```python
from build123d import *

# Parameters (mm, degrees)
BOSS_EXTRUDE1_DEPTH      = 9
BOSS_EXTRUDE1_DEPTH_BACK = 9
SKETCH1_R                = 1.625
SKETCH2_OUTSIDE_W        = 79.846
SKETCH2_OUTSIDE_H        = 80.774
SKETCH2_OUTSIDE_R        = 3
CUT_EXTRUDE1_DEPTH       = 19.574175621
CUT_EXTRUDE1_DRAFT       = -60
SKETCH3_OUTSIDE_W        = 79.846
SKETCH3_OUTSIDE_H        = 80.774
SKETCH3_OUTSIDE_R        = 3
CUT_EXTRUDE2_DEPTH       = 19.574175621
CUT_EXTRUDE2_DRAFT       = -60
CHAMFER1_SIZE            = 0.25


with BuildPart() as part:
    # Sketch1 → Boss-Extrude1 (new, two sides: drawn at the far end of the back side and taken through both)
    with BuildSketch(Plane.XY.offset(-BOSS_EXTRUDE1_DEPTH_BACK)):
        Polygon((0, 3.464101615), (-3, 1.732050808), (-3, -1.732050808), (0, -3.464101615), (3, -1.732050808), (3, 1.732050808), align=None)
        Circle(SKETCH1_R, mode=Mode.SUBTRACT)
    extrude(amount=BOSS_EXTRUDE1_DEPTH + BOSS_EXTRUDE1_DEPTH_BACK)


with BuildPart() as cut_extrude1_tool:
    # Sketch2 outside → Cut-Extrude1 (with draft: the straight prism first)
    with BuildSketch(Plane(origin=(0, 0, -9), x_dir=(-1, 0, 0), z_dir=(0, 0, -1))):
        Rectangle(SKETCH2_OUTSIDE_W, SKETCH2_OUTSIDE_H)
        Circle(SKETCH2_OUTSIDE_R, mode=Mode.SUBTRACT)
    extrude(amount=-CUT_EXTRUDE1_DEPTH)
    # Cut-Extrude1: the draft: its side faces are tilted about the plane it starts from
    cut_extrude1_sides = [cut_extrude1_tool.faces().sort_by_distance(p)[0] for p in [
        (0, -40.387, 0.787087811),
        (-39.923, 0, 0.787087811),
        (0, 40.387, 0.787087811),
        (39.923, 0, 0.787087811),
        (3, 0, 0.787087811),
    ]]
    draft(cut_extrude1_sides, Plane(origin=(0, 0, -9), x_dir=(-1, 0, 0), z_dir=(0, 0, -1)), CUT_EXTRUDE1_DRAFT)


with BuildPart() as part_1:
    add(part.part)

    # Cut-Extrude1: cut by cut_extrude1_tool
    add(cut_extrude1_tool.part, mode=Mode.SUBTRACT)


with BuildPart() as cut_extrude2_tool:
    # Sketch3 outside → Cut-Extrude2 (with draft: the straight prism first)
    with BuildSketch(Plane.XY.offset(9)):
        Rectangle(SKETCH3_OUTSIDE_W, SKETCH3_OUTSIDE_H)
        Circle(SKETCH3_OUTSIDE_R, mode=Mode.SUBTRACT)
    extrude(amount=-CUT_EXTRUDE2_DEPTH)
    # Cut-Extrude2: the draft: its side faces are tilted about the plane it starts from
    cut_extrude2_sides = [cut_extrude2_tool.faces().sort_by_distance(p)[0] for p in [
        (0, -40.387, -0.787087811),
        (39.923, 0, -0.787087811),
        (0, 40.387, -0.787087811),
        (-39.923, 0, -0.787087811),
        (-3, 0, -0.787087811),
    ]]
    draft(cut_extrude2_sides, Plane.XY.offset(9), CUT_EXTRUDE2_DRAFT)


with BuildPart() as part_2:
    add(part_1.part)

    # Cut-Extrude2: cut by cut_extrude2_tool
    add(cut_extrude2_tool.part, mode=Mode.SUBTRACT)

    # Chamfer1
    chamfer1_edges = [part_2.edges().sort_by_distance(p)[0] for p in [
        (-1.625, 0, -9),
        (-1.625, 0, 9),
    ]]
    chamfer(chamfer1_edges, length=CHAMFER1_SIZE)


solid = part_2.part
```
For this review, take the finished solid that the model builds, in its own axes (mm). Round coordinates to 2 decimals unless told otherwise and drop trailing zeros. Order: outer loops, then holes, each group sorted by start corner. A loop starts at its lowest first (then second) coordinate and runs counter-clockwise, first axis right, second up.
Q1. Insertion check: P1, Ø2.5, axis at x = 0, y = 0, coming from the +Z side. The pin has a flat end and moves straight along its axis. Give the tip position at first contact, or say it passes through.
Findings below:
P1: passes through
Q2. Wall thickness on line 1 (Y direction, x = -0.75, z = 0.5); line 2 (X direction, y = 0.5, z = 2.25); line 3 (Y direction, x = 0.5, z = -2.25): over which ranges is each line inside the solid? List them lowest first.
Findings below:
line 1: y = -3.03 to -1.44, 1.44 to 3.03
line 2: x = -3 to -1.55, 1.55 to 3
line 3: y = -3.18 to -1.55, 1.55 to 3.18
Q3. We need section A-A, the plane z = 2.75. Give the boundary of the cut face in (x, y) (3 decimals), plus the area to 3 significant figures.
Findings below:
outline: (-3, -1.732) - (0, -3.464) - (3, -1.732) - (3, 1.732) - (0, 3.464) - (-3, 1.732) - close; hole circle Ø3.25 at (0, 0)
area: 22.9 mm2
